Geometry check sheet. Reference: the model listing, model coordinates, mm. Face numbers are marked on the shaded views. A direction names the side the tool comes from. Give positions to 0.01 mm unless a question says otherwise; leave off trailing zeros. Loops run counter-clockwise (first coordinate to the right, second up) from the corner with the lowest first, then second, coordinate; pieces in that order, holes last. Notation, with made-up numbers: (39, 45) -> (71, 45) arc R30 ccw to (71, 83) -> close; hole circle Ø1 at (35.25, 71). An arc over 180 degrees is marked (long way). Write item = value, one per line.
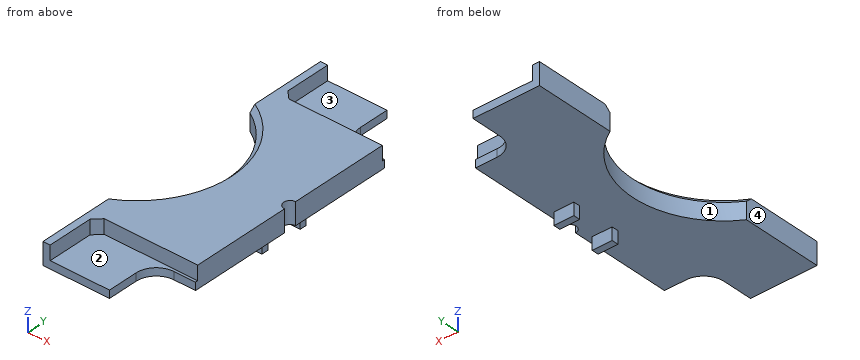
```python
from build123d import *

# Parameters (mm, degrees)
SKETCH_W        = 21.5
SKETCH_H        = 62.95
PAD_DEPTH       = 4.36
SKETCH001_W     = 3.96
SKETCH001_H     = 1.33
PAD001_DEPTH    = 2.46
SKETCH002_W     = 40.406182
SKETCH002_H     = 15.340348
POCKET_DEPTH    = 2.84
CHAMFER_SIZE    = 1.5
CHAMFER001_SIZE = 1.5
SKETCH003_R     = 1.25
POCKET001_DEPTH = 6.821
SKETCH004_R     = 17.85
POCKET002_DEPTH = 5
CHAMFER002_SIZE = 1
SKETCH005_W     = 26.6657
SKETCH005_H     = 14.870099
POCKET003_DEPTH = 5
FILLET_R        = 4
FILLET001_R     = 4


with BuildPart() as part:
    # Sketch → Pad (new body)
    with BuildSketch(Plane.XY):
        Rectangle(SKETCH_W, SKETCH_H)
    extrude(amount=PAD_DEPTH)

    # Sketch001 → Pad001 (join)
    with BuildSketch(Plane.XY):
        with Locations((7.57, 4.335)):
            Rectangle(SKETCH001_W, SKETCH001_H)
    pad001 = extrude(amount=-PAD001_DEPTH)

    # Mirrored: Pad001 across Sketch001 H_Axis
    add(pad001.mirror(Plane.ZX))

    # Sketch002 (on Face5 of Mirrored) → Pocket (cut)
    with BuildSketch(Plane.XY.offset(4.36)):
        with Locations((10.883091, 28.620174)):
            Rectangle(SKETCH002_W, SKETCH002_H)
    pocket = extrude(amount=-POCKET_DEPTH, mode=Mode.SUBTRACT)

    # Chamfer
    chamfer_edges = [part.edges().sort_by_distance(p)[0] for p in [
        (-9.32, 20.95, 2.94),
    ]]
    chamfer(chamfer_edges, length=CHAMFER_SIZE)

    # Mirrored001: Pocket across Sketch002 H_Axis
    add(pocket.mirror(Plane(origin=(0, 0, 4.36), x_dir=(0, 0, 1), z_dir=(0, 1, 0))), mode=Mode.SUBTRACT)

    # Chamfer001
    chamfer001_edges = [part.edges().sort_by_distance(p)[0] for p in [
        (-9.32, -20.95, 2.94),
    ]]
    chamfer(chamfer001_edges, length=CHAMFER001_SIZE)

    # Sketch003 (on Face1 of Chamfer001) → Pocket001 (cut, through all)
    with BuildSketch(Plane.XY.offset(4.36)):
        with Locations((10.75, 0)):
            Circle(SKETCH003_R)
    extrude(amount=-POCKET001_DEPTH, mode=Mode.SUBTRACT)

    # Sketch004 (on Face1 of Pocket001) → Pocket002 (cut)
    with BuildSketch(Plane.XY.offset(4.36)):
        with Locations((-19.675, 0)):
            Circle(SKETCH004_R)
    extrude(amount=-POCKET002_DEPTH, mode=Mode.SUBTRACT)

    # Chamfer002
    chamfer002_edges = [part.edges().sort_by_distance(p)[0] for p in [
        (-4.216447, 8.925, 4.36),
        (-4.216447, -8.925, 4.36),
    ]]
    chamfer(chamfer002_edges, length=CHAMFER002_SIZE)

    # Sketch005 (on Face19 of Chamfer002) → Pocket003 (cut)
    with BuildSketch(Plane.XY.offset(1.52)):
        with Locations((15.78285, 28.88505)):
            Rectangle(SKETCH005_W, SKETCH005_H)
    pocket003 = extrude(amount=-POCKET003_DEPTH, mode=Mode.SUBTRACT)

    # Fillet
    fillet_edges = [part.edges().sort_by_distance(p)[0] for p in [
        (2.45, 21.45, 0.76),
    ]]
    fillet(fillet_edges, radius=FILLET_R)

    # Mirrored002: Pocket003 across Sketch005 H_Axis
    add(pocket003.mirror(Plane(origin=(0, 0, 1.52), x_dir=(0, 0, 1), z_dir=(0, 1, 0))), mode=Mode.SUBTRACT)

    # Fillet001
    fillet001_edges = [part.edges().sort_by_distance(p)[0] for p in [
        (2.45, -21.45, 0.76),
    ]]
    fillet(fillet001_edges, radius=FILLET001_R)


solid = part.part
```
Item 1: Section check B-B, the plane x = 7.25. Record the cut outline in (y, z).
Answer:
outline = (-21.45, 0) -> (-5, 0) -> (-5, -2.46) -> (-3.67, -2.46) -> (-3.67, 0) -> (3.67, 0) -> (3.67, -2.46) -> (5, -2.46) -> (5, 0) -> (21.45, 0) -> (21.45, 1.52) -> (20.95, 1.52) -> (20.95, 4.36) -> (-20.95, 4.36) -> (-20.95, 1.52) -> (-21.45, 1.52) -> close
Item 2: Section check A-A, the plane z = -0.75. Record the cut outline in (x, y), plus the area to 3 significant figures.
Answer:
outline = (5.59, -5) -> (9.55, -5) -> (9.55, -3.67) -> (5.59, -3.67) -> close; (5.59, 3.67) -> (9.55, 3.67) -> (9.55, 5) -> (5.59, 5) -> close
area = 10.5 mm^2
Item 3: Section check C-C, the plane y = 0. Record the cut outline in (x, z) (3 decimals).
Answer:
outline = (-1.825, 0) -> (9.5, 0) -> (9.5, 4.36) -> (-0.825, 4.36) -> (-1.825, 3.36) -> close
Item 4: Gauge pin test, flat ends, axial feed: pin 1 (0.5 mm diameter, centred on y = -29.5, z = 1, fed in from +X); pin 2 (5 mm diameter, centred on x = -4, y = -8, fed in from -Z); pin 3 (0.7 mm diameter, centred on y = 4, z = -1.5, fed in from +X). Record the tip position at first contact, or that the pin passes through.
Answer:
pin_1 = 2.45
pin_2 = 0
pin_3 = 9.55
Item 5: Draft check along Y on the marked faces 1 and 2. Enter one of: +Y half, -Y half, draft (parallel to the pull), parting line (faces both ways), or undercut.
Answer:
face_1 = undercut
face_2 = draft
Item 6: Thickness scan on L1, parallel to Y at x = -5.25, z = 3.5; L2, parallel to Y at x = 7.5, z = -1.5; L3, parallel to Z at x = -5.75, y = 28.5. Record the ranges inside material, lowest first. Write a range as [from, to].
Answer:
L1 = [-20.95, -10.75], [10.75, 20.95]
L2 = [-5, -3.67], [3.67, 5]
L3 = [0, 1.52]
Item 7: Tool access check on the marked faces 3 and 4. Record the directions out of +Z, -Z, +X, -X, +Y, -Y that give a thin tool (end or side, any length) a straight path to the whole face; none if there is none.
Answer:
face_3 = +Z, +X, +Y
face_4 = +Z, -Z, -X, +Y, -Y
Item 8: Section check D-D, the plane y = -23. Record the cut outline in (x, z), plus the area to 3 significant figures.
Answer:
outline = (-10.75, 0) -> (3.29, 0) -> (3.29, 1.52) -> (-9.32, 1.52) -> (-9.32, 4.36) -> (-10.75, 4.36) -> close
area = 25.4 mm^2
